from build123d import *

# Parameters (mm, degrees)
SKETCH1_R           = 5
BOSS_EXTRUDE1_DEPTH = 100
FILLET3_R           = 2
SKETCH2_R           = 6
BOSS_EXTRUDE2_DEPTH = 20
SKETCH3_R           = 2
CUT_EXTRUDE2_DEPTH  = 20


with BuildPart() as part:
    # Sketch1 → Boss-Extrude1 (new body)
    with BuildSketch(Plane.XY):
        Circle(SKETCH1_R)
    extrude(amount=BOSS_EXTRUDE1_DEPTH)

    # Fillet3
    fillet3_edges = [part.edges().sort_by_distance(p)[0] for p in [
        (-5, 0, 0),
    ]]
    fillet(fillet3_edges, radius=FILLET3_R)

    # Sketch2 → Boss-Extrude2 (add)
    with BuildSketch(Plane.XY.offset(100)):
        Circle(SKETCH2_R)
    extrude(amount=BOSS_EXTRUDE2_DEPTH)

    # Sketch3 → Cut-Extrude2 (cut)
    with BuildSketch(Plane.XY.offset(120)):
        with Locations((-2, 0)):
            Circle(SKETCH3_R)
        with Locations((2.1, 0)):
            Circle(SKETCH3_R)
    extrude(amount=-CUT_EXTRUDE2_DEPTH, mode=Mode.SUBTRACT)


solid = part.part
Design review of the part built by this model. Coordinates are the model's own, in mm. A direction names the side the tool comes from. Round coordinates to 2 decimals unless told otherwise and drop trailing zeros. Write each loop counter-clockwise with the first axis right and the second up, starting at its lowest first coordinate (ties: lowest second). Pieces come first, ordered by that corner, then holes. Notation, with made-up numbers: (7.25, 9.25) -> (45.25, 9.25) arc R21 cw to (45.25, 19.25) -> close; hole circle Ø7 at (88.25, 8). An arc over 180 degrees is marked (long way). One line per item, written item: value. Start each with the question number.
Q1. The part is to be moulded in two halves that separate along X. For faces 4 (the face through (-1.08, -4.88, 50.31)), 5 (the face through (0, -1, 120)), 6 (the face through (2, 0, 100)), say which applies: pulls with the +X half, pulls with the -X half, needs draft (parallel to the pull), parting line crosses it, or undercut.
Q2. Insertion check: P1, Ø5, axis at y = -1, z = 78.5, coming from the +X side; P2, Ø6.5, axis at x = 2.1, y = 0, coming from the -Z side; P3, Ø6, axis at x = 4.5, z = 73, coming from the -Y side; P4, Ø5, axis at y = -1, z = 33, coming from the -X side. Each pin has a flat end and moves straight along its axis. Give the tip position at first contact, or say it passes through.
Q3. Tool access review of faces 1 (the face through (-4, 4, 100)), 2 (the face through (1.666, -1.952, 110.14)), 3 (the face through (-6, 0, 110)): name each direction out of +Z, -Z, +X, -X, +Y, -Y from which nothing blocks a thin tool from reaching the whole face with its end or side.
Q4. Add section B-B (z = 84.5). Give the boundary of the cut face in (x, y).
Q5. To check wall thickness, follow probe 1 along Z at (x, y) = (5, -1.25); probe 2 along Y at (x, z) = (2.5, 107); probe 3 along Y at (x, z) = (-2, 110). State the ranges of each line that lie inside material, in increasing order.
Q6. Add section A-A (y = 0). Give the boundary of the cut face in (x, z), then the cut area to 3 significant figures.
Response:
1. face 4: parting line crosses it
1. face 5: needs draft
1. face 6: undercut
2. P1: stops at x = 5
2. P2: stops at z = 0
2. P3: stops at y = -4.77
2. P4: stops at x = -5
3. face 1: -Z
3. face 2: +Z
3. face 3: +Z, -Z
4. outline: circle Ø10 at (0, 0)
5. probe 1: z = 100 to 120
5. probe 2: y = -5.45 to -1.96, 1.96 to 5.45
5. probe 3: y = -5.66 to -2, 2 to 5.66
6. outline: (-6, 100) -> (-5, 100) -> (-5, 2) arc R2 ccw to (-3, 0) -> (3, 0) arc R2 ccw to (5, 2) -> (5, 100) -> (6, 100) -> (6, 120) -> (4.1, 120) -> (4.1, 100) -> (0.1, 100) -> (0.1, 120) -> (0, 120) -> (0, 100) -> (-4, 100) -> (-4, 120) -> (-6, 120) -> close
6. area: 1,080 mm^2
